The listing builds one solid part. Answer for the finished solid, in the listing's coordinates (mm). A direction names the side the tool comes from. Coordinates: 2 decimals unless noted, no trailing zeros. Loops run counter-clockwise (first coordinate to the right, second up) from the corner with the lowest first, then second, coordinate; pieces in that order, holes last. Notation, with made-up numbers: (78.25, 37.5) - (84.25, 37.5) arc R29 cw to (84.25, 75.5) - close; hole circle Ø10 at (-18.75, 11). An arc over 180 degrees is marked (long way). Write each question's results on one line, items separated by ' | '. Start each with the question number.
(1) Determine the mould class of faces 4 (the flat face through (61, 25, 29)), 5 (the flat face through (54, 0, 7.5)), 6 (the flat face through (49, 0, 12.5)) for opening direction Y: released by +Y, released by -Y, zero draft, split by the parting line, or undercut.
(2) Find section B-B on z = 25. Determine the outline of the cut face in (x, y), then the cut area to 3 significant figures.
(3) Find section C-C on x = 62.5. Determine the outline of the cut face in (y, z), then the cut area to 3 significant figures.
(4) Given pin 1 Ø7 at (x, y) = (51.5, -4.5) entering from -Z; pin 2 Ø1.5 at (y, z) = (3.5, 3.5) entering from -X; pin 3 Ø1 at (x, y) = (-5, 16) entering from -Z; pin 4 Ø2 at (x, y) = (54, 12) entering from -Z, each flat-ended and moving along its own axis, determine where each tip first touches the part or whether it passes through.
(5) Find section A-A on x = -20. Determine the outline of the cut face in (y, z).
(6) Find section D-D on y = -15. Determine the outline of the cut face in (x, z).
(7) For faces 1 (the flat face through (68, 0, 42.5)), 2 (the flat face through (27, 0, 5)), 3 (the flat face through (-1, -30, 25)), determine the directions among +Z, -Z, +X, -X, +Y, -Y from which every point of the face is accessible in a straight line to the end or side of a thin tool.
(8) Consider line 1 (X direction, y = 27.5, z = 25); line 2 (Z direction, x = -20, y = 28.1); line 3 (Z direction, x = 14.5, y = -12.5). Determine where each line is inside the solid, lowest interval first. Write a range as from..to.
from build123d import *

# Parameters (mm, degrees)
SKETCH2_W               = 100
SKETCH2_H               = 60
BOSS_EXTRUDE1_DEPTH     = 50
SHELL1_T                = -5
SKETCH4_W               = 60
SKETCH4_H               = 50
CUT_EXTRUDE1_DEPTH      = 10
CUT_EXTRUDE2_DEPTH      = 90.582364336
CUT_EXTRUDE2_DEPTH_BACK = 90.582364336
SKETCH5_R               = 5
BOSS_EXTRUDE2_DEPTH     = 60
SKETCH15_W              = 5
SKETCH15_H              = 50
CUT_EXTRUDE4_DEPTH      = 37.5
SHELL3_START            = -20
SHELL3_DEPTH            = 40


# Read off the part's stored shape, not the designer's step: Shell3
with BuildPart() as part:
    # Sketch2 → Boss-Extrude1 (new body)
    with BuildSketch(Plane.XY):
        Rectangle(SKETCH2_W, SKETCH2_H)
    extrude(amount=BOSS_EXTRUDE1_DEPTH)

    # Shell1
    shell1_openings = [part.faces().sort_by_distance(p)[0] for p in [
        (-50, 0, 25),
    ]]
    offset(amount=SHELL1_T, openings=shell1_openings, kind=Kind.INTERSECTION)

    # Sketch4 → Cut-Extrude1 (cut)
    with BuildSketch(Plane.XY.offset(5)):
        with Locations((-20, 0)):
            Rectangle(SKETCH4_W, SKETCH4_H)
    extrude(amount=-CUT_EXTRUDE1_DEPTH, mode=Mode.SUBTRACT)

    # Sketch5 → Cut-Extrude2 (cut, two sides: drawn at the far end of the back side and taken through both)
    with BuildSketch(Plane(origin=(0, -25, 0), x_dir=(1, 0, 0), z_dir=(0, 1, 0)).offset(-CUT_EXTRUDE2_DEPTH_BACK)):
        with Locations(Location((-20, -25, 0), (0, 0, 270))):
            Circle(SKETCH5_R)
    extrude(amount=CUT_EXTRUDE2_DEPTH + CUT_EXTRUDE2_DEPTH_BACK, mode=Mode.SUBTRACT)

    # Sketch13 → Boss-Extrude2 (add)
    with BuildSketch(Plane(origin=(0, 30, 0), x_dir=(1, 0, 0), z_dir=(0, 1, 0))):
        with BuildLine():
            Line((50, -42.5), (57.5, -42.5))
            Line((57.5, -42.5), (87.5, -42.5))
            ThreePointArc((87.5, -42.5), (67.096938471, -29.631195597), (57.5, -7.5))
            Line((57.5, -7.5), (50, -7.5))
            Line((50, -7.5), (50, -42.5))
        make_face()
    extrude(amount=-BOSS_EXTRUDE2_DEPTH)

    # Sketch15 → Cut-Extrude4 (cut)
    with BuildSketch(Plane.YZ.offset(87.5)):
        with Locations((-27.5, 25)):
            Rectangle(SKETCH15_W, SKETCH15_H)
        with Locations((27.5, 25)):
            Rectangle(SKETCH15_W, SKETCH15_H)
    extrude(amount=-CUT_EXTRUDE4_DEPTH, mode=Mode.SUBTRACT)

    # Shell3 outline → Shell3 (cut)
    with BuildSketch(Plane(origin=(0, 0, 0), x_dir=(1, 0, 0), z_dir=(0, 1, 0)).offset(SHELL3_START)):
        with BuildLine():
            Line((53.243409838, -12.5), (45, -12.5))
            Line((45, -12.5), (45, -37.5))
            Line((45, -37.5), (67.860272771, -37.5))
            ThreePointArc((67.860272771, -37.5), (58.527827688, -26.183389184), (53.243409838, -12.5))
        make_face()
    extrude(amount=SHELL3_DEPTH, mode=Mode.SUBTRACT)


solid = part.part
Values:
1) face 4: released by +Y | face 5: zero draft | face 6: undercut
2) outline: (-50, -30) - (-25, -30) - (-25, -25) - (-50, -25) - close; (-50, 25) - (-25, 25) - (-25, 30) - (-50, 30) - close; (-15, -30) - (50, -30) - (50, -25) - (63.66, -25) - (63.66, 25) - (50, 25) - (50, 30) - (-15, 30) - (-15, 25) - (45, 25) - (45, 20) - (57.86, 20) - (57.86, -20) - (45, -20) - (45, -25) - (-15, -25) - close | area: 1,320 mm²
3) outline: (-25, 23.06) - (25, 23.06) - (25, 42.5) - (-25, 42.5) - close; hole (-20, 31.92) - (20, 31.92) - (20, 37.5) - (-20, 37.5) - close | area: 749 mm²
4) pin 1: stops at z = 0 | pin 2: stops at x = 10 | pin 3: stops at z = 45 | pin 4: stops at z = 7.5
5) outline: (-30, 0) - (-25, 0) - (-25, 20) - (-30, 20) - close; (-30, 30) - (-25, 30) - (-25, 45) - (25, 45) - (25, 30) - (30, 30) - (30, 50) - (-30, 50) - close; (25, 0) - (30, 0) - (30, 20) - (25, 20) - close
6) outline: (-50, 45) - (45, 45) - (45, 37.5) - (67.86, 37.5) arc R45.88 ccw to (53.24, 12.5) - (45, 12.5) - (45, 5) - (10, 5) - (10, 0) - (50, 0) - (50, 7.5) - (57.5, 7.5) arc R40.88 cw to (87.5, 42.5) - (50, 42.5) - (50, 50) - (-50, 50) - close
7) face 1: +Z, +X, +Y, -Y | face 2: -X | face 3: +Z, -Z, +X, -X, -Y
8) line 1: x = -50..-25, -15..50 | line 2: z = 0..20, 30..50 | line 3: z = 0..5, 45..50
